Autodesk Inventor part; units mm, degrees
ref_plane "YZ Plane" through (0, 0, 0) normal (1, 0, 0) x (0, 1, 0)
ref_plane "XZ Plane" through (0, 0, 0) normal (0, 1, 0) x (-1, 0, 0)
ref_plane "XY Plane" through (0, 0, 0) normal (0, 0, 1) x (1, 0, 0)
sketch "Sketch1" plane through (0, 0, 0) normal (1, 0, 0) x (0, 1, 0)
  line L0 (0, 0) -> (25.4, 0)
  line L1 (25.4, 0) -> (25.4, -50.8)
  line L2 (25.4, -50.8) -> (0, -50.8)
  line L3 (0, -50.8) -> (0, 0)
  line L4 (23.8125, -1.5875) -> (1.5875, -1.5875)
  line L5 (1.5875, -1.5875) -> (1.5875, -49.2125)
  line L6 (1.5875, -49.2125) -> (23.8125, -49.2125)
  line L7 (23.8125, -49.2125) -> (23.8125, -1.5875)
  dimension "d0" = 25.4
  dimension "d1" = 50.8
  dimension "d2" = 1.5875
extrude "Extrusion1" add sketch "Sketch1" along normal blind 241.3
sketch "Sketch2" plane through (0, 25.4, 0) normal (0, 1, 0) x (1, 0, 0)
  line L0 (0, 50.8) -> (0, 0)
  line L1 (0, 0) -> (241.3, 0)
  line L2 (241.3, 50.8) -> (241.3, 0)
  line L3 (0, 50.8) -> (241.3, 50.8)
  circle A0 centre (12.7, 25.4) radius 2.5781
  circle A1 centre (228.6, 25.4) radius 2.5781
  point P0 (0, 0)
  dimension "d5" = 5.1562
  dimension "d6" = 12.7
  dimension "d7" = 5.1562
  dimension "d8" = 12.7
  dimension "d9" = 25.4
  dimension "d10" = 25.4
extrude "Extrusion2" cut sketch "Sketch2" against normal blind 25.4 contours A0 | A1
sketch "Sketch4" plane through (0, 0, 0) normal (0, 0, 1) x (1, 0, 0)
  line L0 (0, 25.4) -> (0, 0)
  line L1 (0, 0) -> (241.3, 0)
  line L2 (241.3, 25.4) -> (241.3, 0)
  line L3 (0, 25.4) -> (241.3, 25.4)
  line L4 (120.65, 25.4) -> (120.65, 0) construction
  circle A0 centre (107.95, 12.7) radius 2.5781
  circle A1 centre (133.35, 12.7) radius 2.5781
  dimension "d21" = 5.1562
  dimension "d22" = 5.1562
  dimension "d23" = 12.7
  dimension "d24" = 25.4
  dimension "d27" = 12.7
  dimension "d28" = 12.7
extrude "Extrusion4" cut sketch "Sketch4" against normal through all contours A0 | A1
properties part number "2inTubeBase"
Geometry check sheet. Reference: the model listing, model coordinates, mm. A direction names the side the tool comes from. Round coordinates to 2 decimals unless told otherwise and drop trailing zeros. Order: outer loops, then holes, each group sorted by start corner. A loop starts at its lowest first (then second) coordinate and runs counter-clockwise, first axis right, second up. Notation, with made-up numbers: M 28.25,67.25 L 64.25,67.25 A15 ccw 64.25,71.25 Z; hole C 39,-39 d4. An arc over 180 degrees is marked long. Answer in a Markdown table with one row per item.
(1) Scan lines: probe 1 along X at (y, z) = (24.2, -25.4); probe 2 along Z at (x, y) = (92, 17.75); probe 3 along Z at (x, y) = (12.7, 24.85). Record each from-to range of solid material in increasing order. Write a range as from..to.
Responses:
| item | result |
|---|---|
| probe 1 | x = 0..10.12, 15.28..226.02, 231.18..241.3 |
| probe 2 | z = -50.8..-49.21, -1.59..0 |
| probe 3 | z = -50.8..-27.98, -22.82..0 |
(2) Tool access check on faces 4 (the face through (119, 23.812, -26)), 5 (the face through (135.8, 13.5, -0.8)). Record the directions out of +Z, -Z, +X, -X, +Y, -Y that give a thin tool (end or side, any length) a straight path to the whole face; none if there is none.
Responses:
| item | result |
|---|---|
| face 4 | +X, -X |
| face 5 | +Z, -Z |
(3) Go/stop test with a flat-tipped pin: P1, Ø3, axis at x = 228.6, z = -25.4, coming from the -Y side. Record where the tip stops, or that it passes through.
Responses:
| item | result |
|---|---|
| P1 | passes through |
(4) Sectioned sample at C-C, the plane y = 20.75. Record the cut outline in (x, z).
Responses:
| item | result |
|---|---|
| outline | M 0,-50.8 L 241.3,-50.8 L 241.3,-49.21 L 0,-49.21 Z; M 0,-1.59 L 241.3,-1.59 L 241.3,0 L 0,0 Z |
(5) Draft check along Y on faces 1 (the face through (119, 13, -50.8)), 2 (the face through (119, 25.4, -25)), 3 (the face through (110.33, 11.71, -0.78)). Enter one of: released by +Y, released by -Y, zero draft, split by the parting line, or undercut.
Responses:
| item | result |
|---|---|
| face 1 | zero draft |
| face 2 | released by +Y |
| face 3 | undercut |
(6) Sectioned sample at A-A, the plane x = 12.7. Record the cut outline in (y, z).
Responses:
| item | result |
|---|---|
| outline | M 0,-50.8 L 25.4,-50.8 L 25.4,-27.98 L 23.81,-27.98 L 23.81,-49.21 L 1.59,-49.21 L 1.59,-27.98 L 0,-27.98 Z; M 0,-22.82 L 1.59,-22.82 L 1.59,-1.59 L 23.81,-1.59 L 23.81,-22.82 L 25.4,-22.82 L 25.4,0 L 0,0 Z |
(7) Sectioned sample at B-B, the plane z = -41. Record the cut outline in (x, y).
Responses:
| item | result |
|---|---|
| outline | M 0,0 L 241.3,0 L 241.3,1.59 L 0,1.59 Z; M 0,23.81 L 241.3,23.81 L 241.3,25.4 L 0,25.4 Z |
(8) Sectioned sample at D-D, the plane z = -25.4. Record the cut outline in (x, y).
Responses:
| item | result |
|---|---|
| outline | M 0,0 L 10.12,0 L 10.12,1.59 L 0,1.59 Z; M 0,23.81 L 10.12,23.81 L 10.12,25.4 L 0,25.4 Z; M 15.28,0 L 226.02,0 L 226.02,1.59 L 15.28,1.59 Z; M 15.28,23.81 L 226.02,23.81 L 226.02,25.4 L 15.28,25.4 Z; M 231.18,0 L 241.3,0 L 241.3,1.59 L 231.18,1.59 Z; M 231.18,23.81 L 241.3,23.81 L 241.3,25.4 L 231.18,25.4 Z |
